For this review, take the finished solid that the model builds, in its own axes (mm). A direction names the side the tool comes from. Round coordinates to 2 decimals unless told otherwise and drop trailing zeros. Order: outer loops, then holes, each group sorted by start corner. A loop starts at its lowest first (then second) coordinate and runs counter-clockwise, first axis right, second up. Notation, with made-up numbers: (21.5, -4.75) - (77.5, -4.75) arc R20 cw to (77.5, 22.25) - close; hole circle Ø3 at (87, -26.75). An arc over 180 degrees is marked (long way). Write each question's results on one line, items separated by ' | '. Start each with the question number.
(1) Insertion check: pin 1 Ø3 at (x, y) = (-2.5, 4) entering from +Z; pin 2 Ø3 at (y, z) = (4, -12) entering from -X; pin 3 Ø1.9 at (y, z) = (4, -7) entering from -X. Each pin has a flat end and moves straight along its axis. Give the tip position at first contact, or say it passes through.
(2) For L1, parallel to X at y = 1, z = -11; L2, parallel to X at y = 5.75, z = -0.75; L3, parallel to Z at x = -5.5, y = 5.5, list the stretches that pass through material, from the lowest coordinate up. Write a range as from..to.
(3) Take a section at A-A, the plane z = 4. Give the boundary of the cut face in (x, y), plus the area to 3 significant figures.
(4) Take a section at C-C, the plane y = 2.5. Give the boundary of the cut face in (x, z).
(5) Draft analysis for pull direction X (two halves, no side actions). For faces 1 (the flat face through (0, 5, -5.4)), 2 (the flat face through (-0.999, 5, -7)), 3 (the cylindrical face through (0.12, 4.93, -14.154)), state which applies: pulls with the +X half, pulls with the -X half, needs draft (parallel to the pull), parting line crosses it, or undercut.
(6) Take a section at D-D, the plane x = -1.75. Give the boundary of the cut face in (y, z), plus the area to 3 significant figures.
(7) Take a section at B-B, the plane x = 0. Give the boundary of the cut face in (y, z), plus the area to 3 significant figures.
(8) For faces 4 (the flat face through (-4, 5, -5.9)), 5 (the flat face through (5.95, 5, 0)), 6 (the flat face through (0.999, 5, -7)), 7 (the flat face through (-5.95, 5, 0)), list the 3-axis set-ups (+Z, -Z, +X, -X, +Y, -Y) from which the entire face can be reached by the end or side of a thin tool; tool diameter is ignored.
```python
from build123d import *

# Parameters (mm, degrees)
SKETCH3_W           = 12.9
SKETCH3_H           = 11.8
BOSS_EXTRUDE2_DEPTH = 10
SKETCH4_W           = 11.9
SKETCH4_H           = 10.8
CUT_EXTRUDE1_DEPTH  = 10
SKETCH5_W           = 11.3990209
SKETCH5_H           = 5.9
CUT_EXTRUDE2_DEPTH  = 10
SKETCH6_W           = 1.998577766
SKETCH6_H           = 2.842465616
BOSS_EXTRUDE3_DEPTH = 10
SKETCH7_R           = 3.054866119
BOSS_EXTRUDE4_DEPTH = 10
SKETCH8_R           = 2.006377858
CUT_EXTRUDE3_DEPTH  = 10


with BuildPart() as part:
    # Sketch3 → Boss-Extrude2 (new body)
    with BuildSketch(Plane(origin=(0, 0, 0), x_dir=(1, 0, 0), z_dir=(0, 1, 0))):
        Rectangle(SKETCH3_W, SKETCH3_H)
    extrude(amount=BOSS_EXTRUDE2_DEPTH)

    # Sketch4 → Cut-Extrude1 (cut)
    with BuildSketch(Plane(origin=(0, 0, 0), x_dir=(1, 0, 0), z_dir=(0, 1, 0))):
        Rectangle(SKETCH4_W, SKETCH4_H)
    extrude(amount=CUT_EXTRUDE1_DEPTH, mode=Mode.SUBTRACT)

    # Sketch5 → Cut-Extrude2 (cut)
    with BuildSketch(Plane(origin=(0, 0, 0), x_dir=(1, 0, 0), z_dir=(0, 1, 0))):
        with Locations((0.25048955, -2.95)):
            Rectangle(SKETCH5_W, SKETCH5_H)
    extrude(amount=CUT_EXTRUDE2_DEPTH, mode=Mode.SUBTRACT)

    # Sketch6 → Boss-Extrude3 (add)
    with BuildSketch(Plane(origin=(0, 0, 0), x_dir=(1, 0, 0), z_dir=(0, 1, 0))):
        with Locations((0, 6.821232808)):
            Rectangle(SKETCH6_W, SKETCH6_H)
    extrude(amount=BOSS_EXTRUDE3_DEPTH)

    # Sketch7 → Boss-Extrude4 (add)
    with BuildSketch(Plane(origin=(0, 0, 0), x_dir=(1, 0, 0), z_dir=(0, 1, 0))):
        with Locations((0, 11.101611726)):
            Circle(SKETCH7_R)
    extrude(amount=BOSS_EXTRUDE4_DEPTH)

    # Sketch8 → Cut-Extrude3 (cut)
    with BuildSketch(Plane(origin=(0, 0, 0), x_dir=(1, 0, 0), z_dir=(0, 1, 0))):
        with Locations(Location((0, 11.101611726, 0), (0, 0, 270))):
            Circle(SKETCH8_R)
    extrude(amount=CUT_EXTRUDE3_DEPTH, mode=Mode.SUBTRACT)


solid = part.part
```
Results below:
1) pin 1: stops at z = -5.4 | pin 2: stops at x = -3.05 | pin 3: stops at x = -1
2) L1: x = -3.05..-2, 2..3.05 | L2: x = -6.45..-5.95, 5.95..6.45 | L3: z = -5.9..-5.4, 5.4..5.9
3) outline: (-6.45, 0) - (-5.95, 0) - (-5.95, 10) - (-6.45, 10) - close; (5.95, 0) - (6.45, 0) - (6.45, 10) - (5.95, 10) - close | area: 10.0 mm^2
4) outline: (-6.45, -5.9) - (-1, -5.9) - (-1, -8.21) arc R3.05 ccw (long way) to (1, -8.21) - (1, -5.9) - (6.45, -5.9) - (6.45, 5.9) - (5.95, 5.9) - (5.95, -5.4) - (-5.95, -5.4) - (-5.95, 5.4) - (-5.45, 5.4) - (-5.45, 5.9) - (-6.45, 5.9) - close; hole circle Ø4.01 at (0, -11.1)
5) face 1: undercut | face 2: pulls with the -X half | face 3: parting line crosses it
6) outline: (0, -13.61) - (10, -13.61) - (10, -12.08) - (0, -12.08) - close; (0, -10.12) - (10, -10.12) - (10, -8.6) - (0, -8.6) - close; (0, -5.9) - (10, -5.9) - (10, -5.4) - (0, -5.4) - close | area: 35.5 mm^2
7) outline: (0, -14.16) - (10, -14.16) - (10, -13.11) - (0, -13.11) - close; (0, -9.1) - (10, -9.1) - (10, -5.4) - (0, -5.4) - close | area: 47.4 mm^2
8) face 4: -X, +Y, -Y | face 5: +Z, +Y, -Y | face 6: +X, +Y, -Y | face 7: +Y, -Y
